Could you check a few things on this drawing? It's one solid part, dimensions in mm from its lowest x, y, z. Give positions to 0.01 mm unless a question says otherwise; leave off trailing zeros. Order: outer loops, then holes, each group sorted by start corner. A loop starts at its lowest first (then second) coordinate and runs counter-clockwise, first axis right, second up.
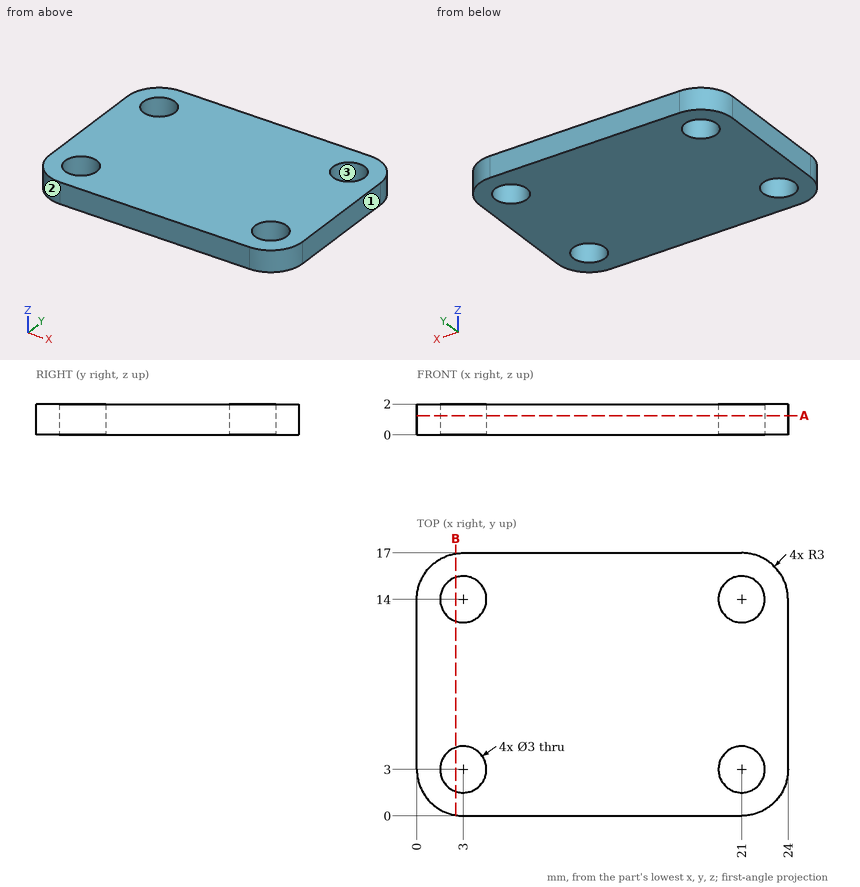
Item 1: Please list where these lines run through material, in increasing order: line 1 along Y through (x, z) = (3, 0.5); line 2 along X through (y, z) = (3.25, 0.85); line 3 along X through (y, z) = (13.25, 1.25).
Findings:
line 1: y = 0 to 1.5, 4.5 to 12.5, 15.5 to 17
line 2: x = 0 to 1.52, 4.48 to 19.52, 22.48 to 24
line 3: x = 0 to 1.7, 4.3 to 19.7, 22.3 to 24
Item 2: We'd pull the mould along Y, two halves only. Please class the marked faces 1, 2 and 3: +Y half, -Y half, draft (parallel to the pull), parting line (faces both ways), or undercut.
Findings:
face 1: draft
face 2: -Y half
face 3: undercut
Item 3: Imagine slicing it at B-B on x = 2.5. List the corners of the cut face in (y, z) for me.
Findings:
outline: (0.04, 0) - (1.59, 0) - (1.59, 2) - (0.04, 2) - close; (4.41, 0) - (12.59, 0) - (12.59, 2) - (4.41, 2) - close; (15.41, 0) - (16.96, 0) - (16.96, 2) - (15.41, 2) - close
Item 4: Imagine slicing it at A-A on z = 1.25. List the corners of the cut face in (x, y) for me, then the cut area to 3 significant figures.
Findings:
outline: (0, 3) arc R3 ccw to (3, 0) - (21, 0) arc R3 ccw to (24, 3) - (24, 14) arc R3 ccw to (21, 17) - (3, 17) arc R3 ccw to (0, 14) - close; hole circle Ø3 at (3, 3); hole circle Ø3 at (3, 14); hole circle Ø3 at (21, 3); hole circle Ø3 at (21, 14)
area: 372 mm2
